Input: part model. Units: mm. Frame: model coordinates. A direction names the side the tool comes from. Coordinates: 2 decimals unless noted, no trailing zeros. Loops run counter-clockwise (first coordinate to the right, second up) from the corner with the lowest first, then second, coordinate; pieces in that order, holes last.
(1) Mould query, pull axis Y, two halves, no side actions, for faces 1 (the face through (0, 0, 10)), 2 (the face through (-19.33, 0.85, 20.85)), 3 (the face through (-11, -14, 33)). Classes: released by +Y, released by -Y, zero draft, split by the parting line, or undercut.
(2) Section B-B, the plane z = 25. Return loops of the section in (x, y).
(3) Section A-A, the plane y = 0. Return loops of the section in (x, z), then the cut area to 3 significant figures.
(4) Contact query for flat-ended pins moving along their axis: P1, Ø2, axis at y = -16, z = 20, coming from the -X side; P2, Ø10, axis at x = 5, z = 20.5, coming from the +Y side; P3, Ø3, axis at x = -10, y = 21.5, coming from the +Z side; P4, Ø10, axis at x = 22, y = 0.5, coming from the -Z side. Output: stop coordinate, or through.
(5) Line query: L1, parallel to Y at x = 0, z = 23; L2, parallel to Z at x = 20.5, y = -5. Output: solid intervals per line, ascending.
(6) Set-up query: faces 4 (the face through (0, 0, 0)), 5 (the face through (19, -6, 10)). Return all of +Z, -Z, +X, -X, +Y, -Y with unobstructed straight access to the full face (end or side cutting, diameter ignored); none if empty.
```python
from build123d import *

# Parameters (mm, degrees)
F0_R     = 29.35
F0_R_2   = 19.35
F0_R_3   = 17.35
F1_DEPTH = 10
F2_SIZE  = 4
F3_DEPTH = 33
F4_R     = 1


with BuildPart() as f1:
    # F0 (on Top) → F1 (new body)
    with BuildSketch(Plane.XY):
        Circle(F0_R)
        Circle(F0_R_2, mode=Mode.SUBTRACT)
        Circle(F0_R_2)
        Circle(F0_R_3, mode=Mode.SUBTRACT)
        Circle(F0_R_3)
    extrude(amount=F1_DEPTH)

    # F2
    f2_edges = [f1.edges().sort_by_distance(p)[0] for p in [
        (-29.35, 0, 0),
    ]]
    chamfer(f2_edges, length=F2_SIZE)

    # F0 (on Top) → F3 (join)
    with BuildSketch(Plane.XY):
        Circle(F0_R_2)
        Circle(F0_R_3, mode=Mode.SUBTRACT)
    extrude(amount=F3_DEPTH)

    # F4
    f4_edges = [f1.edges().sort_by_distance(p)[0] for p in [
        (-19.35, 0, 33),
    ]]
    fillet(f4_edges, radius=F4_R)


solid = f1.part
```
Report:
1. face 1: undercut
1. face 2: split by the parting line
1. face 3: zero draft
2. outline: circle Ø38.7 at (0, 0); hole circle Ø34.7 at (0, 0)
3. outline: (-29.35, 4) - (-25.35, 0) - (25.35, 0) - (29.35, 4) - (29.35, 10) - (19.35, 10) - (19.35, 32) arc R1 ccw to (18.35, 33) - (17.35, 33) - (17.35, 10) - (-17.35, 10) - (-17.35, 33) - (-18.35, 33) arc R1 ccw to (-19.35, 32) - (-19.35, 10) - (-29.35, 10) - close
3. area: 663 mm2
4. P1: stops at x = -12.22
4. P2: stops at y = 19.35
4. P3: stops at z = 10
4. P4: stops at z = 0
5. L1: y = -19.35 to -17.35, 17.35 to 19.35
5. L2: z = 0 to 10
6. face 4: -Z, +X, -X, +Y, -Y
6. face 5: +Z
